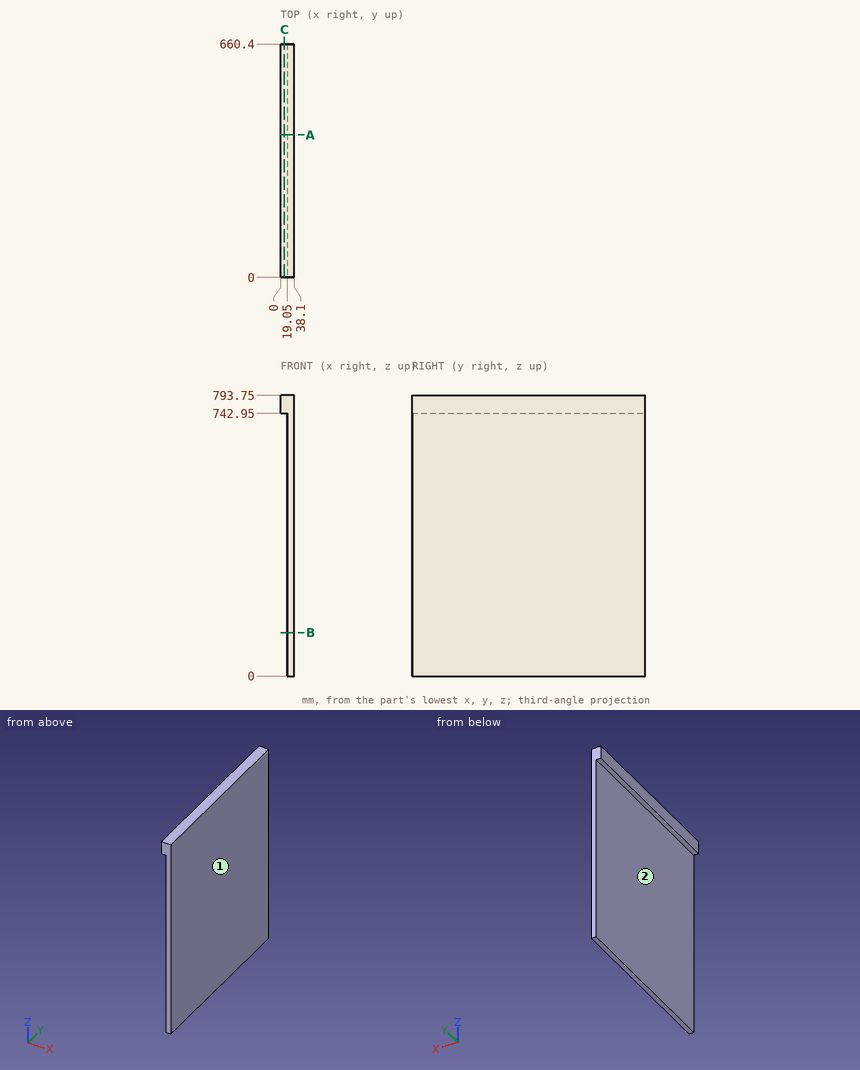
Part print with two shaded views. Sizes in mm from the minimum x, y, z corner. A direction names the side the tool comes from. Round coordinates to 2 decimals unless told otherwise and drop trailing zeros. Loops run counter-clockwise (first coordinate to the right, second up) from the corner with the lowest first, then second, coordinate; pieces in that order, holes last. Notation, with made-up numbers: (-7, -6.75) - (8, -6.75) arc R28 cw to (8, 30.25) - close; hole circle Ø3 at (-4, 60). An arc over 180 degrees is marked (long way). Answer as a JSON object with one key per item and string values.
Item 1: Band-saw the part on B-B on z = 122.5. List the corners of the cut face in (x, y), plus the area to 3 significant figures.
Output:
{"outline": "(19.05, 0) - (38.1, 0) - (38.1, 660.4) - (19.05, 660.4) - close", "area": "12,600 mm2"}
Item 2: Band-saw the part on A-A on y = 403.5. List the corners of the cut face in (x, z).
Output:
{"outline": "(0, 742.95) - (19.05, 742.95) - (19.05, 0) - (38.1, 0) - (38.1, 793.75) - (0, 793.75) - close"}
Item 3: Wall check: L1, parallel to Z at x = 5, y = 547; L2, parallel to X at y = 385, z = 477. Give the ranges that are in metal, low to high.
Output:
{"L1": "742.95 to 793.75", "L2": "19.05 to 38.1"}
Item 4: Pin check, flat tips, straight feed: pin 1 (10 mm diameter, centred on x = 13.5, z = 439, fed in from -Y); pin 2 (4 mm diameter, centred on y = 419, z = 367.5, fed in from -X); pin 3 (15 mm diameter, centred on x = 10, y = 429, fed in from -Z). Stop position of each tip, or through.
Output:
{"pin 1": "through", "pin 2": "x = 19.05", "pin 3": "z = 742.95"}
Item 5: Band-saw the part on C-C on x = 11. List the corners of the cut face in (y, z).
Output:
{"outline": "(0, 742.95) - (660.4, 742.95) - (660.4, 793.75) - (0, 793.75) - close"}
Item 6: Tool access for the marked faces 1 and 2: list every direction of +Z, -Z, +X, -X, +Y, -Y with a clear straight run to the whole face (end or side of a thin tool).
Output:
{"face 1": "+Z, -Z, +X, +Y, -Y", "face 2": "-Z, -X, +Y, -Y"}
